from build123d import *

# Parameters (mm, degrees)
SKETCH_1_W          = 116
SKETCH_1_H          = 56
EXTRUDE_1_DEPTH     = 3
SKETCH_2_W          = 93
SKETCH_2_H          = 56
EXTRUDE_2_DEPTH     = 3
SKETCH_3_W          = 93
SKETCH_3_H          = 27
EXTRUDE_3_DEPTH     = 4
SKETCH_5_W          = 12
SKETCH_5_H          = 12
EXTRUDE_4_DEPTH     = 3
SKETCH_6_R          = 2.6
CUT_EXTRUDE_1_DEPTH = 3
CUT_EXTRUDE_2_DEPTH = 74.518705103
SKETCH_8_W          = 70
SKETCH_8_H          = 12
CUT_EXTRUDE_3_DEPTH = 94.364875622
SKETCH_9_W          = 4
SKETCH_9_H          = 3
CUT_EXTRUDE_4_DEPTH = 88.709748603
CUT_EXTRUDE_5_DEPTH = 91.93404203
FILLET_1_R          = 2


with BuildPart() as part:
    # 草图1 → 凸台-拉伸1 (new body)
    with BuildSketch(Plane(origin=(0, 0, 0), x_dir=(1, 0, 0), z_dir=(0, 1, 0))):
        Rectangle(SKETCH_1_W, SKETCH_1_H)
    extrude(amount=EXTRUDE_1_DEPTH)

    # 草图2 → 凸台-拉伸2 (add)
    with BuildSketch(Plane(origin=(0, 3, 0), x_dir=(1, 0, 0), z_dir=(0, 1, 0))):
        Rectangle(SKETCH_2_W, SKETCH_2_H)
    extrude(amount=EXTRUDE_2_DEPTH)

    # 草图3 → 凸台-拉伸3 (add)
    with BuildSketch(Plane.XY.offset(28)):
        with Locations((0, 13.5)):
            Rectangle(SKETCH_3_W, SKETCH_3_H)
    extrude(amount=EXTRUDE_3_DEPTH)

    # 草图5 → 凸台-拉伸4 (add)
    with BuildSketch(Plane(origin=(0, 3, 0), x_dir=(1, 0, 0), z_dir=(0, 1, 0))):
        with Locations((48, 34)):
            Rectangle(SKETCH_5_W, SKETCH_5_H)
        with Locations((-48, 34)):
            Rectangle(SKETCH_5_W, SKETCH_5_H)
    extrude(amount=-EXTRUDE_4_DEPTH)

    # 草图6 → 切除-拉伸1 (cut)
    with BuildSketch(Plane(origin=(0, 3, 0), x_dir=(1, 0, 0), z_dir=(0, 1, 0))):
        with Locations(Location((-48, 34, 0), (0, 0, 270))):
            Circle(SKETCH_6_R)
        with Locations(Location((48, 34, 0), (0, 0, 270))):
            Circle(SKETCH_6_R)
    extrude(amount=-CUT_EXTRUDE_1_DEPTH, mode=Mode.SUBTRACT)

    # 草图7 → 切除-拉伸2 (cut, through all)
    with BuildSketch(Plane(origin=(0, 6, 0), x_dir=(1, 0, 0), z_dir=(0, 1, 0))):
        Polygon((-18.64631219, 18), (0, 5.160153957), (18.64631219, 18), align=None)
        Polygon((-8.5, 0), (-38.5, 17.320508076), (-38.5, -17.320508076), align=None)
        Polygon((38.5, -17.320508076), (8.5, 0), (38.5, 17.320508076), align=None)
        Polygon((-18.64631219, -18), (18.64631219, -18), (0, -5.160153957), align=None)
    extrude(amount=-CUT_EXTRUDE_2_DEPTH, mode=Mode.SUBTRACT)

    # 草图8 → 切除-拉伸3 (cut, through all)
    with BuildSketch(Plane(origin=(0, 0, 28), x_dir=(-1, 0, 0), z_dir=(0, 0, -1))):
        with Locations((0, 16.5)):
            Rectangle(SKETCH_8_W, SKETCH_8_H)
    extrude(amount=-CUT_EXTRUDE_3_DEPTH, mode=Mode.SUBTRACT)

    # 草图9 → 切除-拉伸4 (cut, through all)
    with BuildSketch(Plane(origin=(0, 0, -28), x_dir=(-1, 0, 0), z_dir=(0, 0, -1))):
        with Locations((56, 1.5)):
            Rectangle(SKETCH_9_W, SKETCH_9_H)
        with Locations((-56, 1.5)):
            Rectangle(SKETCH_9_W, SKETCH_9_H)
    extrude(amount=-CUT_EXTRUDE_4_DEPTH, mode=Mode.SUBTRACT)

    # 草图10 → 切除-拉伸5 (cut, through all)
    with BuildSketch(Plane(origin=(0, 0, 28), x_dir=(-1, 0, 0), z_dir=(0, 0, -1))):
        with BuildLine():
            Line((-46.5, 20.7), (-42.5, 20.7))
            ThreePointArc((-42.5, 20.7), (-40.3, 18.5), (-42.5, 16.3))
            Line((-42.5, 16.3), (-46.5, 16.3))
            ThreePointArc((-46.5, 16.3), (-48.7, 18.5), (-46.5, 20.7))
        make_face()
        with BuildLine():
            Line((46.5, 20.7), (42.5, 20.7))
            ThreePointArc((42.5, 20.7), (40.3, 18.5), (42.5, 16.3))
            Line((42.5, 16.3), (46.5, 16.3))
            ThreePointArc((46.5, 16.3), (48.7, 18.5), (46.5, 20.7))
        make_face()
    extrude(amount=-CUT_EXTRUDE_5_DEPTH, mode=Mode.SUBTRACT)

    # 圆角1
    fillet_1_edges = [part.edges().sort_by_distance(p)[0] for p in [
        (0, 3, -5.160153957),
        (-18.64631219, 3, -18),
        (-18.64631219, 3, 18),
        (0, 3, 5.160153957),
        (18.64631219, 3, 18),
        (-8.5, 3, 0),
        (-38.5, 3, 17.320508076),
        (-38.5, 3, -17.320508076),
        (-35, 22.5, 30),
        (-35, 10.5, 30),
        (35, 10.5, 30),
        (35, 22.5, 30),
        (38.5, 3, -17.320508076),
        (38.5, 3, 17.320508076),
        (8.5, 3, 0),
        (18.64631219, 3, -18),
    ]]
    fillet(fillet_1_edges, radius=FILLET_1_R)


solid = part.part
Could you check a few things on this model? Use its own coordinates, in mm. A direction names the side the tool comes from. Give positions to 0.01 mm unless a question says otherwise; leave off trailing zeros. Write each loop counter-clockwise with the first axis right and the second up, starting at its lowest first coordinate (ties: lowest second). Pieces come first, ordered by that corner, then holes. Notation, with made-up numbers: (10, 11.25) -> (28, 11.25) arc R16 cw to (28, 22.25) -> close; hole circle Ø4 at (12.25, 1.25). An arc over 180 degrees is marked (long way). Write each question's results on one line, items separated by ' | '. Start each with the question number.
Q1. Suppose I cut it at D-D, the plane y = 4.75. List the corners of the cut face in (x, z) for me.
Q2. I'm going to push flat-ended pins straight in: pin 1 Ø4 at (x, y) = (-39, 15) entering from -Z; pin 2 Ø3 at (x, y) = (-4.5, 3) entering from -Z; pin 3 Ø12 at (y, z) = (9.5, -26.5) entering from +X. Where does each tip first touch, or does it pass through?
Q3. We'd pull the mould along Z, two halves only. Please class faces 5 (the face through (-37.475, 2.958, -15.603)), 6 (the face through (46.5, 24, 30)), 7 (the face through (14.114, 2.958, -16.628)): +Z half, -Z half, draft (parallel to the pull), parting line (faces both ways), or undercut.
Q4. Suppose I cut it at A-A, the plane y = 18.5. List the corners of the cut face in (x, z) for me, and give its area (3 significant figures).
Q5. Suppose I cut it at C-C, the plane z = -34. List the corners of the cut face in (x, y) for me, and give its area (3 significant figures).
Q6. Which directions (+Z, -Z, +X, -X, +Y, -Y) give clear straight access to the entire face, cutting with the end or side of a thin tool? Please do faces 1 (the face through (-34.4, 21.93, 30.03)), 2 (the face through (-1, 6, 0)), 3 (the face through (-45, 20.7, 30)), 4 (the face through (-23.67, 3.04, 8.76)).
Q7. Suppose I cut it at B-B, the plane x = 48. List the corners of the cut face in (y, z) for me, and give its area (3 significant figures).
Q8. I need wall thicknesses on probe 1 along X at (y, z) = (1.75, -34); probe 2 along X at (y, z) = (1.5, 0.5); probe 3 along X at (y, z) = (3.5, 9). Which ranges of each line are inside material? Lowest first, please.
Outcome:
1) outline: (-46.5, -28) -> (46.5, -28) -> (46.5, 32) -> (-46.5, 32) -> close; hole (-38.5, -13.86) arc R2 ccw to (-35.5, -15.59) -> (-11.5, -1.73) arc R2 ccw to (-11.5, 1.73) -> (-35.5, 15.59) arc R2 ccw to (-38.5, 13.86) -> close; hole (-13.35, -14.35) arc R2 ccw to (-12.22, -18) -> (12.22, -18) arc R2 ccw to (13.35, -14.35) -> (1.13, -5.94) arc R2 ccw to (-1.13, -5.94) -> close; hole (-13.35, 14.35) -> (-1.13, 5.94) arc R2 ccw to (1.13, 5.94) -> (13.35, 14.35) arc R2 ccw to (12.22, 18) -> (-12.22, 18) arc R2 ccw to start; hole (11.5, -1.73) -> (35.5, -15.59) arc R2 ccw to (38.5, -13.86) -> (38.5, 13.86) arc R2 ccw to (35.5, 15.59) -> (11.5, 1.73) arc R2 ccw to start
2) pin 1: z = 28 | pin 2: z = -28 | pin 3: x = 46.5
3) face 5: undercut | face 6: draft | face 7: undercut
4) outline: (-40.3, 28) -> (-35, 28) -> (-35, 32) -> (-40.3, 32) -> close; (35, 28) -> (40.3, 28) -> (40.3, 32) -> (35, 32) -> close | area: 42.4 mm2
5) outline: (-54, 0) -> (-50.6, 0) -> (-50.6, 3) -> (-54, 3) -> close; (-45.4, 0) -> (-42, 0) -> (-42, 3) -> (-45.4, 3) -> close; (42, 0) -> (45.4, 0) -> (45.4, 3) -> (42, 3) -> close; (50.6, 0) -> (54, 0) -> (54, 3) -> (50.6, 3) -> close | area: 40.8 mm2
6) face 1: +Z, -Z | face 2: -Z, +X, -X, +Y | face 3: +Z, -Z, -X | face 4: +Y, -Y
7) outline: (0, -40) -> (3, -40) -> (3, -36.6) -> (0, -36.6) -> close; (0, -31.4) -> (3, -31.4) -> (3, 28) -> (0, 28) -> close | area: 188 mm2
8) probe 1: -54 to -50.6, -45.4 to -42, 42 to 45.4, 50.6 to 54 | probe 2: -54 to -38.5, -10.56 to 10.56, 38.5 to 54 | probe 3: -46.5 to -38.5, -24.09 to -5.58, 5.58 to 24.09, 38.5 to 46.5
